from build123d import *

# Parameters (mm, degrees)
F0_W     = 102.187556
F0_H     = 18.34783
F1_DEPTH = 94.996
F2_W     = 98.708875
F2_H     = 20.189193
F3_DEPTH = 112.776


with BuildPart() as f1:
    # F0 (on Top) → F1 (new body)
    with BuildSketch(Plane.XY):
        with Locations((-14.888035, 9.173915)):
            Rectangle(F0_W, F0_H)
    extrude(amount=-F1_DEPTH)

    # F2 (on Front) → F3 (join)
    with BuildSketch(Plane.XZ):
        with Locations((-17.250094, -40.75765)):
            Rectangle(F2_W, F2_H)
    extrude(amount=F3_DEPTH)


solid = f1.part
CAD build for the part. Positions are in the model's coordinates, mm. A direction names the side the tool comes from. Round coordinates to 2 decimals unless told otherwise and drop trailing zeros. Write each loop counter-clockwise with the first axis right and the second up, starting at its lowest first coordinate (ties: lowest second). Pieces come first, ordered by that corner, then holes.
(1) Slice it at D-D, the plane z = -69. Write the cut outline in (x, y).
(2) Slice it at A-A, the plane z = -47. Write the cut outline in (x, y), and give its area (3 significant figures).
(3) Probe line 1 along Y through (x, z) = (-39, -16.5); line 2 along X through (y, z) = (-2.5, -38); line 3 along Z through (x, y) = (-59.5, -45). List the from-to ranges inside material, lowest first.
(4) Slice it at B-B, the plane x = -16.5. Write the cut outline in (y, z), and give its area (3 significant figures).
(5) Slice it at C-C, the plane y = -39.5. Write the cut outline in (x, z), and give its area (3 significant figures).
(6) Drop flat-ended pins along their axis: P1, Ø6, axis at x = -55, y = -40.5, coming from the -Z side; P2, Ø1, axis at x = -4, z = -23, coming from the -Y side; P3, Ø12, axis at y = -30, z = -58, coming from the +X side; P4, Ø10, axis at y = -73, z = -43.5, coming from the +X side. Give the stop position or say it passes through.
(7) 3-axis set-ups, long thin cutter, end or side, ignore diameter. For faces 1 (the face through (-65.982, 9, -47)), 2 (the face through (-18, -56, -30.663)), 3 (the face through (32.104, -56, -41)), 4 (the face through (-18, -56, -50.852)): which of +Z, -Z, +X, -X, +Y, -Y reach the whole face in a straight line?
From the geometry:
1. outline: (-65.98, 0) - (36.21, 0) - (36.21, 18.35) - (-65.98, 18.35) - close
2. outline: (-66.6, -112.78) - (32.1, -112.78) - (32.1, 0) - (36.21, 0) - (36.21, 18.35) - (-65.98, 18.35) - (-65.98, 0) - (-66.6, 0) - close
2. area: 13,000 mm2
3. line 1: y = 0 to 18.35
3. line 2: x = -66.6 to 32.1
3. line 3: z = -50.85 to -30.66
4. outline: (-112.78, -50.85) - (0, -50.85) - (0, -95) - (18.35, -95) - (18.35, 0) - (0, 0) - (0, -30.66) - (-112.78, -30.66) - close
4. area: 4,020 mm2
5. outline: (-66.6, -50.85) - (32.1, -50.85) - (32.1, -30.66) - (-66.6, -30.66) - close
5. area: 1,990 mm2
6. P1: stops at z = -50.85
6. P2: stops at y = 0
6. P3: passes through
6. P4: stops at x = 32.1
7. face 1: +Z, -Z, -X, +Y
7. face 2: +Z, +X, -X, -Y
7. face 3: +Z, -Z, +X, -Y
7. face 4: -Z, +X, -X, -Y
